Input: part model. Units: mm. Frame: model coordinates. Coordinates: 2 decimals unless noted, no trailing zeros. Loops run counter-clockwise (first coordinate to the right, second up) from the corner with the lowest first, then second, coordinate; pieces in that order, holes last. Notation, with made-up numbers: M 5.5,70.5 L 43.5,70.5 A28 cw 43.5,89.5 Z; hole C 18.25,27 d7. An arc over 180 degrees is marked long. Use a Markdown table: item, result. Add a question column.
1. Line query: L1, parallel to Y at x = 49.5, z = 3.45; L2, parallel to Y at x = 6.5, z = 3.15; L3, parallel to X at y = 66, z = 0.55. Output: solid intervals per line, ascending. Write a range as [from, to].
2. Pin query (flat end, axial travel): pin 1 (1.5 mm diameter, centred on y = 41.5, z = 2.5, fed in from +X); pin 2 (2 mm diameter, centred on x = 56, z = 1.5, fed in from -Y); pin 3 (1.5 mm diameter, centred on y = 30.5, z = 2.5, fed in from +X). Return the tip coordinate at first contact, or that it passes through.
3. Section A-A on z = 3.2. Output: boundary loops of the cut face in (x, y), then the cut area to 3 significant figures.
4. Draft query along X for faces 1 (the flat face through (23.575, 47.631, 1.972)), 2 (the flat face through (66.5, 60, 2)), 3 (the cylindrical face through (8, 5, 2)). Return one class per face: +X half, -X half, draft (parallel to the pull), parting line (faces both ways), or undercut.
5. Section B-B on x = 6.5. Output: boundary loops of the cut face in (y, z), then the cut area to 3 significant figures.
6. Section D-D on y = 55. Output: boundary loops of the cut face in (x, z).
7. Section C-C on y = 5. Output: boundary loops of the cut face in (x, z), then the cut area to 3 significant figures.
```python
from build123d import *

# Parameters (mm, degrees)
SKETCH_1_R      = 1.5
EXTRUDE_1_DEPTH = 4


with BuildPart() as part:
    # 草图1 → 凸台-拉伸1 (new body)
    with BuildSketch(Plane.XY):
        Polygon((0, 0), (13, 0), (66.5, 45.5), (66.5, 74.5), (46.5, 74.5), (0, 20), align=None)
        with Locations((6.5, 15)):
            Circle(SKETCH_1_R, mode=Mode.SUBTRACT)
        with Locations(Location((6.5, 5, 0), (0, 0, 180))):
            Circle(SKETCH_1_R, mode=Mode.SUBTRACT)
        with Locations((49, 55)):
            Circle(SKETCH_1_R, mode=Mode.SUBTRACT)
        with Locations(Location((64, 55, 0), (0, 0, 180))):
            Circle(SKETCH_1_R, mode=Mode.SUBTRACT)
        with Locations(Location((49, 65, 0), (0, 0, 180))):
            Circle(SKETCH_1_R, mode=Mode.SUBTRACT)
        with Locations((64, 65)):
            Circle(SKETCH_1_R, mode=Mode.SUBTRACT)
    extrude(amount=EXTRUDE_1_DEPTH)


solid = part.part
```
Answers below:
| question | item | result |
|---|---|---|
| 1 | L1 | y = [31.04, 53.59], [56.41, 63.59], [66.41, 74.5] |
| 1 | L2 | y = [0, 3.5], [6.5, 13.5], [16.5, 27.62] |
| 1 | L3 | x = [39.25, 47.88], [50.12, 62.88], [65.12, 66.5] |
| 2 | pin 1 | stops at x = 62.68 |
| 2 | pin 2 | stops at y = 35.72 |
| 2 | pin 3 | stops at x = 49.74 |
| 3 | outline | M 0,0 L 13,0 L 66.5,45.5 L 66.5,74.5 L 46.5,74.5 L 0,20 Z; hole C 6.5,5 d3; hole C 6.5,15 d3; hole C 49,55 d3; hole C 49,65 d3; hole C 64,55 d3; hole C 64,65 d3 |
| 3 | area | 2,430 mm² |
| 4 | face 1 | -X half |
| 4 | face 2 | +X half |
| 4 | face 3 | undercut |
| 5 | outline | M 0,0 L 3.5,0 L 3.5,4 L 0,4 Z; M 6.5,0 L 13.5,0 L 13.5,4 L 6.5,4 Z; M 16.5,0 L 27.62,0 L 27.62,4 L 16.5,4 Z |
| 5 | area | 86.5 mm² |
| 6 | outline | M 29.86,0 L 47.5,0 L 47.5,4 L 29.86,4 Z; M 50.5,0 L 62.5,0 L 62.5,4 L 50.5,4 Z; M 65.5,0 L 66.5,0 L 66.5,4 L 65.5,4 Z |
| 7 | outline | M 0,0 L 5,0 L 5,4 L 0,4 Z; M 8,0 L 18.88,0 L 18.88,4 L 8,4 Z |
| 7 | area | 63.5 mm² |
